Build history of the part. All positions in model axes, mm. Face numbers are marked on the shaded views. A direction names the side the tool comes from. Coordinates: 2 decimals unless noted, no trailing zeros. Order: outer loops, then holes, each group sorted by start corner. A loop starts at its lowest first (then second) coordinate and runs counter-clockwise, first axis right, second up. Notation, with made-up numbers: (-17, -5.5) - (1, -5.5) arc R15 ccw to (1, 4.5) - close; hole circle Ø11 at (85, -37.75). An arc over 180 degrees is marked (long way). Write each question's results on one line, items separated by ' | '.
from build123d import *

# Parameters (mm, degrees)
CYLINDER_R              = 10
CYLINDER_DEPTH          = 10
CYLINDER001_R           = 2
CYLINDER001_DEPTH       = 30
CYLINDER001_ROLL_ANGLE  = -90
PAD001_DEPTH            = 10
CYLINDER002_R           = 4
CYLINDER002_DEPTH       = 12
CYLINDER002_PITCH_ANGLE = 90
BOX002_W                = 10
BOX002_H                = 2.5
BOX002_DEPTH            = 10
BOX003_W                = 10
BOX003_H                = 2.5
BOX003_DEPTH            = 10
PAD_DEPTH               = 2.5
BOX004_W                = 10
BOX004_H                = 10
BOX004_DEPTH            = 5
BOX005_W                = 10
BOX005_H                = 10
BOX005_DEPTH            = 5
BOX001_W                = 15
BOX001_H                = 10
BOX001_DEPTH            = 10
CYLINDER003_R           = 6
CYLINDER003_DEPTH       = 2
CYLINDER003_PITCH_ANGLE = 90
BOX_W                   = 40
BOX_H                   = 30
BOX_DEPTH               = 10


with BuildPart() as cylinder:
    # Cylinder → Cylinder (new body)
    with BuildSketch(Plane.XY.offset(-5)):
        Circle(CYLINDER_R)
    extrude(amount=CYLINDER_DEPTH)


with BuildPart() as cylinder001:
    # Cylinder001 → Cylinder001 (new body)
    with BuildSketch(Plane.XY):
        Circle(CYLINDER001_R)
    extrude(amount=CYLINDER001_DEPTH)


with BuildPart() as cylinder001_1:
    # Cylinder001 roll: moved
    add(cylinder001.part.rotate(Axis((0, 0, 0), (1, 0, 0)), CYLINDER001_ROLL_ANGLE))


with BuildPart() as cylinder001_2:
    # Cylinder001 placement: moved
    add(cylinder001_1.part.moved(Location((-15, -15, 0))))


with BuildPart() as other_nut:
    # Sketch001 → Pad001 (new body)
    with BuildSketch(Plane.YZ):
        Polygon((3.464102, 6), (-3.464102, 6), (-6.928203, 0), (-3.464102, -6), (3.464102, -6), (6.928203, 0), align=None)
    extrude(amount=-PAD001_DEPTH)


with BuildPart() as other_nut_1:
    # Body001 placement: moved
    add(other_nut.part.moved(Location((15, 0, 0))))


with BuildPart() as other_screw:
    # Cylinder002 → Cylinder002 (new body)
    with BuildSketch(Plane.XY):
        Circle(CYLINDER002_R)
    extrude(amount=CYLINDER002_DEPTH)


with BuildPart() as other_screw_1:
    # Cylinder002 pitch: moved
    add(other_screw.part.rotate(Axis((0, 0, 0), (0, 1, 0)), CYLINDER002_PITCH_ANGLE))


with BuildPart() as other_screw_2:
    # Cylinder002 placement: moved
    add(other_screw_1.part.moved(Location((10, 0, 0))))


with BuildPart() as cube002:
    # Box002 → Box002 (new body)
    with BuildSketch(Plane(origin=(-20, 12.5, -5), x_dir=(1, 0, 0), z_dir=(0, 0, 1))):
        with Locations((5, 1.25)):
            Rectangle(BOX002_W, BOX002_H)
    extrude(amount=BOX002_DEPTH)


with BuildPart() as cube003:
    # Box003 → Box003 (new body)
    with BuildSketch(Plane(origin=(-20, -15, -5), x_dir=(1, 0, 0), z_dir=(0, 0, 1))):
        with Locations((5, 1.25)):
            Rectangle(BOX003_W, BOX003_H)
    extrude(amount=BOX003_DEPTH)


with BuildPart() as body:
    # Sketch → Pad (new body)
    with BuildSketch(Plane.XZ):
        Polygon((0, -4.041452), (3.5, -2.020726), (3.5, 2.020726), (0, 4.041452), (-3.5, 2.020726), (-3.5, -2.020726), align=None)
    extrude(amount=-PAD_DEPTH)


with BuildPart() as body_1:
    # Body placement: moved
    add(body.part.moved(Location((-15, -12.5, 0))))


with BuildPart() as cube004:
    # Box004 → Box004 (new body)
    with BuildSketch(Plane(origin=(15, -5, -10), x_dir=(1, 0, 0), z_dir=(0, 0, 1))):
        with Locations((5, 5)):
            Rectangle(BOX004_W, BOX004_H)
    extrude(amount=BOX004_DEPTH)


with BuildPart() as cube005:
    # Box005 → Box005 (new body)
    with BuildSketch(Plane(origin=(15, -5, 5), x_dir=(1, 0, 0), z_dir=(0, 0, 1))):
        with Locations((5, 5)):
            Rectangle(BOX005_W, BOX005_H)
    extrude(amount=BOX005_DEPTH)


with BuildPart() as negative_fusion:
    # Box001 → Box001 (new body)
    with BuildSketch(Plane(origin=(-20, -5, -5), x_dir=(1, 0, 0), z_dir=(0, 0, 1))):
        with Locations((7.5, 5)):
            Rectangle(BOX001_W, BOX001_H)
    extrude(amount=BOX001_DEPTH)

    # Fusion: union Cylinder, Cylinder001, Other Nut, Other Screw, Cube002, Cube003, Body, Cube004, Cube005
    add(cylinder.part)
    add(cylinder001_2.part)
    add(other_nut_1.part)
    add(other_screw_2.part)
    add(cube002.part)
    add(cube003.part)
    add(body_1.part)
    add(cube004.part)
    add(cube005.part)


with BuildPart() as cylinder002:
    # Cylinder003 → Cylinder003 (new body)
    with BuildSketch(Plane.XY):
        Circle(CYLINDER003_R)
    extrude(amount=CYLINDER003_DEPTH)


with BuildPart() as cylinder002_1:
    # Cylinder003 pitch: moved
    add(cylinder002.part.rotate(Axis((0, 0, 0), (0, 1, 0)), CYLINDER003_PITCH_ANGLE))


with BuildPart() as cylinder002_2:
    # Cylinder003 placement: moved
    add(cylinder002_1.part.moved(Location((20, 0, 0))))


with BuildPart() as cut:
    # Box → Box (new body)
    with BuildSketch(Plane(origin=(-20, -15, -5), x_dir=(1, 0, 0), z_dir=(0, 0, 1))):
        with Locations((20, 15)):
            Rectangle(BOX_W, BOX_H)
    extrude(amount=BOX_DEPTH)

    # Fusion001: union Cylinder002
    add(cylinder002_2.part)

    # Cut: cut Negative Fusion
    add(negative_fusion.part, mode=Mode.SUBTRACT)


solid = cut.part
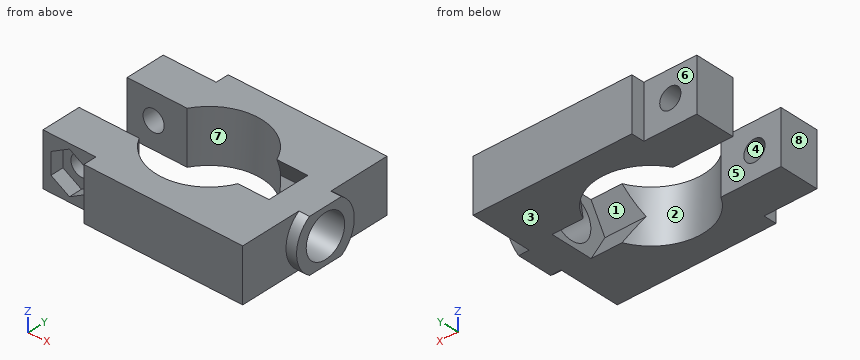
1. Tool access for the marked faces 1, 2, 3, 4 and 5: list every direction of +Z, -Z, +X, -X, +Y, -Y with a clear straight run to the whole face (end or side of a thin tool).
Solved:
face 1: none | face 2: +Z, -Z | face 3: -Z, +X, -X, +Y, -Y | face 4: +Y, -Y | face 5: +Z, -Z, -X
2. Band-saw the part on B-B on y = 0. Give the cut face in (x, z).
Solved:
outline: (15, -5) - (22, -5) - (22, -4) - (15, -4) - close; (15, 4) - (22, 4) - (22, 5) - (15, 5) - close
3. Probe line 1 (X direction, y = -11.75, z = -1); line 2 (Y direction, x = -8, z = 3.25); line 3 (Y direction, x = 17, z = 2.25). List the from-to ranges inside material, lowest first.
Solved:
line 1: x = -20 to -18.5, -11.5 to 20 | line 2: y = -15 to -6, 6 to 15 | line 3: y = -15 to -3.31, 3.31 to 15
4. Band-saw the part on C-C on z = -3. Give the cut face in (x, y), then the cut area to 3 significant figures.
Solved:
outline: (-20, -12.5) - (-16.8, -12.5) - (-16.8, -10) - (-13.2, -10) - (-13.2, -12.5) - (-10, -12.5) - (-10, -15) - (20, -15) - (20, -5.2) - (22, -5.2) - (22, -2.65) - (15, -2.65) - (15, -5.2) - (8.54, -5.2) arc R10 cw to (-8.66, -5) - (-20, -5) - close; (-20, 5) - (-8.66, 5) arc R10 cw to (8.54, 5.2) - (15, 5.2) - (15, 2.65) - (22, 2.65) - (22, 5.2) - (20, 5.2) - (20, 15) - (-10, 15) - (-10, 12.5) - (-20, 12.5) - close | area: 649 mm2
5. Drop flat-ended pins along their axis: pin 1 Ø5 at (x, z) = (-15, -2) entering from -Y; pin 2 Ø0.8 at (y, z) = (14.5, -0.5) entering from -X; pin 3 Ø3 at (y, z) = (-3, 0) entering from -X. Give the stop position or say it passes through.
Solved:
pin 1: stops at y = -12.5 | pin 2: stops at x = -10 | pin 3: stops at x = 15
6. Band-saw the part on D-D on x = 12.5. Give the cut face in (y, z), then the cut area to 3 significant figures.
Solved:
outline: (-15, -5) - (-4.04, -5) - (-6.93, 0) - (-4.04, 5) - (-15, 5) - close; (4.04, -5) - (15, -5) - (15, 5) - (4.04, 5) - (6.93, 0) - close | area: 190 mm2
7. Two-plate mould, pull along X, no slides. Class the marked faces 6, 7 and 8: +X half, -X half, draft (parallel to the pull), parting line (faces both ways), or undercut.
Solved:
face 6: draft | face 7: undercut | face 8: -X half
8. Band-saw the part on A-A on x = -6. Give the cut face in (y, z).
Solved:
outline: (-15, -5) - (-8, -5) - (-8, 5) - (-15, 5) - close; (8, -5) - (15, -5) - (15, 5) - (8, 5) - close
